Part model, mm, in its own coordinate system. A direction names the side the tool comes from. Coordinates: 2 decimals unless noted, no trailing zeros. Loops run counter-clockwise (first coordinate to the right, second up) from the corner with the lowest first, then second, coordinate; pieces in that order, holes last. Notation, with made-up numbers: (-30.75, 82.25) - (-0.75, 82.25) arc R19 cw to (-0.75, 100.25) - close; hole circle Ø4 at (21.5, -15.75). An arc over 180 degrees is marked (long way). One line per question, with ' | ' between items. Start each with the question number.
from build123d import *

# Parameters (mm, degrees)
F0_R     = 10.9
F1_DEPTH = 3


with BuildPart() as f1:
    # F0 (on Front) → F1 (new body)
    with BuildSketch(Plane.XZ):
        with BuildLine():
            ThreePointArc((-103.010684, 68.484581), (-105.728194, 65.462684), (-107.332646, 61.728723))
            ThreePointArc((-107.332646, 61.728723), (-110.919129, 46.724993), (-109.322923, 31.381365))
            ThreePointArc((-109.322923, 31.381365), (-115.194842, 27.743972), (-121.92824, 26.204033))
            ThreePointArc((-121.92824, 26.204033), (-129.60444, 22.960502), (-133.536128, 15.612961))
            Line((-133.536128, 15.612961), (-135.046402, 5.720314))
            Line((-135.046402, 5.720314), (-125.723981, 2.081926))
            ThreePointArc((-125.723981, 2.081926), (-121.748186, 1.239441), (-117.712255, 1.716926))
            ThreePointArc((-117.712255, 1.716926), (-102.925402, 6.112806), (-90.435534, 15.166975))
            ThreePointArc((-90.435534, 15.166975), (-84.349499, 11.90044), (-79.649174, 6.839116))
            ThreePointArc((-79.649174, 6.839116), (-73.002094, 1.813097), (-64.673093, 2.081926))
            Line((-64.673093, 2.081926), (-55.350671, 5.720314))
            Line((-55.350671, 5.720314), (-56.860946, 15.612961))
            ThreePointArc((-56.860946, 15.612961), (-58.119231, 19.477343), (-60.55071, 22.733819))
            ThreePointArc((-60.55071, 22.733819), (-71.75108, 33.341669), (-85.837154, 39.631129))
            ThreePointArc((-85.837154, 39.631129), (-86.05127, 46.535056), (-84.018197, 53.13632))
            ThreePointArc((-84.018197, 53.13632), (-82.989076, 61.405869), (-87.38639, 68.484581))
            Line((-87.38639, 68.484581), (-95.198537, 74.738841))
            Line((-95.198537, 74.738841), (-103.010684, 68.484581))
        make_face()
        with BuildLine():
            ThreePointArc((-120.621098, 24.712317), (-113.206213, 21.304741), (-110.179299, 13.726489))
            ThreePointArc((-110.179299, 13.726489), (-129.152385, 6.148238), (-120.621098, 24.712317))
        make_face(mode=Mode.SUBTRACT)
        with Locations((-95.198537, 28.726489)):
            Circle(F0_R, mode=Mode.SUBTRACT)
        with BuildLine():
            ThreePointArc((-79.010881, 8.716992), (-71.79419, 24.42051), (-58.217775, 13.726489))
            ThreePointArc((-58.217775, 13.726489), (-66.64136, 3.032468), (-79.010881, 8.716992))
        make_face(mode=Mode.SUBTRACT)
        with BuildLine():
            ThreePointArc((-85.963632, 52.750159), (-105.748038, 61.842259), (-84.198537, 58.726489))
            ThreePointArc((-84.198537, 58.726489), (-84.649035, 55.61072), (-85.963632, 52.750159))
        make_face(mode=Mode.SUBTRACT)
    extrude(amount=F1_DEPTH)


solid = f1.part
1) Pin check, flat tips, straight feed: pin 1 Ø6 at (x, z) = (-78, 63.5) entering from +Y; pin 2 Ø1.5 at (x, y) = (-83.5, -0.5) entering from +Z. Stop position of each tip, or through.
2) Tool access for faces 5 (the cylindrical face through (-103.12, -1.479, 6.017)), 6 (the cylindrical face through (-129.516, -1.479, 23.04)): list every direction of +Z, -Z, +X, -X, +Y, -Y with a clear straight run to the whole face (end or side of a thin tool).
3) Band-saw the part on A-A on z = 19.5. List the corners of the cut face in (x, y), then the cut area to 3 significant figures.
4) Band-saw the part on B-B on x = -97.5. List the corners of the cut face in (y, z), then the cut area to 3 significant figures.
5) Band-saw the part on D-D on x = -112.5. List the corners of the cut face in (y, z), then the cut area to 3 significant figures.
6) Band-saw the part on C-C on z = 49.5. List the corners of the cut face in (x, y).
7) Wall check: line 1 along X through (y, z) = (-2.7, 8); line 2 along Z through (x, y) = (-100, -0.35); line 3 along Z through (x, y) = (-101.5, -0.2). Give the ranges that are in metal, low to high. Write a range as [from, to].
8) Mould opens along X. For faces 1 (the cylindrical face through (-82.964, -1.479, 61.29)), 2 (the flat face through (-99.05, -1.479, 71.655)), 3 (the cylindrical face through (-84.637, -1.479, 55.653)), 4 (the flat face through (-89, 0, 19)) say: +X half, -X half, draft (parallel to the pull), parting line (faces both ways), or undercut.
Values found:
1) pin 1: through | pin 2: z = 64.76
2) face 5: -Z, +Y, -Y | face 6: +Z, -X, +Y, -Y
3) outline: (-132.27, -3) - (-130.54, -3) - (-130.54, 0) - (-132.27, 0) - close; (-111.82, -3) - (-101, -3) - (-101, 0) - (-111.82, 0) - close; (-89.39, -3) - (-78.58, -3) - (-78.58, 0) - (-89.39, 0) - close; (-59.85, -3) - (-58.13, -3) - (-58.13, 0) - (-59.85, 0) - close | area: 75.2 mm²
4) outline: (-3, 9.27) - (0, 9.27) - (0, 18.07) - (-3, 18.07) - close; (-3, 39.38) - (0, 39.38) - (0, 47.97) - (-3, 47.97) - close; (-3, 69.48) - (0, 69.48) - (0, 72.9) - (-3, 72.9) - close | area: 62.4 mm²
5) outline: (-3, 2.65) - (0, 2.65) - (0, 6.97) - (-3, 6.97) - close; (-3, 20.48) - (0, 20.48) - (0, 29.08) - (-3, 29.08) - close | area: 38.7 mm²
6) outline: (-110.65, -3) - (-101.19, -3) - (-101.19, 0) - (-110.65, 0) - close; (-89.21, -3) - (-85.43, -3) - (-85.43, 0) - (-89.21, 0) - close
7) line 1: [-134.7, -130.57], [-111.79, -99.48], [-80.47, -78.61], [-59.83, -55.7] | line 2: [7.69, 18.94], [38.51, 48.83], [68.62, 70.89] | line 3: [6.85, 19.83], [37.62, 49.71], [67.74, 69.69]
8) face 1: +X half | face 2: -X half | face 3: undercut | face 4: draft
